from build123d import *

# Parameters (mm, degrees)
SKETCH1_R               = 12.7
BOSS_EXTRUDE1_DEPTH     = 36.83
SKETCH3_R               = 6.35
CUT_EXTRUDE1_DEPTH      = 18.415
CUT_EXTRUDE2_REACH      = 42.976
SKETCH4_R               = 6
CUT_EXTRUDE3_DEPTH      = 18.415
BOSS_EXTRUDE2_DEPTH     = 18.415
CUT_EXTRUDE6_DEPTH      = 18.415
CUT_EXTRUDE4_REACH      = 42.976
CUT_EXTRUDE4_END_RADIUS = 12.7
SKETCH6_R               = 1.5


with BuildPart() as part:
    # Sketch1 → Boss-Extrude1 (new body)
    with BuildSketch(Plane(origin=(0, 0, 0), x_dir=(1, 0, 0), z_dir=(0, 1, 0))):
        with Locations(Location((0, 0, 0), (0, 0, 270))):
            Circle(SKETCH1_R)
    extrude(amount=BOSS_EXTRUDE1_DEPTH)

    # Sketch3 → Cut-Extrude1 (cut)
    with BuildSketch(Plane(origin=(0, 0, 0), x_dir=(-1, 0, 0), z_dir=(0, -1, 0))):
        with Locations(Location((0, 0, 0), (0, 0, 90))):
            Circle(SKETCH3_R)
    extrude(amount=-CUT_EXTRUDE1_DEPTH, mode=Mode.SUBTRACT)

    # Sketch4 → Cut-Extrude2 (cut, up to next)
    with BuildSketch(Plane(origin=(0, 36.83, 0), x_dir=(1, 0, 0), z_dir=(0, 1, 0)), mode=Mode.PRIVATE) as cut_extrude2_sk1:
        with Locations(Location((0, 0, 0), (0, 0, 270))):
            Circle(SKETCH4_R)
    cut_extrude2_tool1 = extrude(cut_extrude2_sk1.sketch, amount=-CUT_EXTRUDE2_REACH, mode=Mode.PRIVATE) & part.part
    add(cut_extrude2_tool1.solids().sort_by_distance((0, 36.83, 0))[0], mode=Mode.SUBTRACT)

    # Sketch5 → Cut-Extrude3 (cut)
    with BuildSketch(Plane(origin=(0, 36.83, 0), x_dir=(1, 0, 0), z_dir=(0, 1, 0))):
        with BuildLine():
            Line((0, 8.032), (-2.0066, 8.032))
            Line((-2.0066, 8.032), (-2.0066, 5.654516464))
            ThreePointArc((-2.0066, 5.654516464), (0, 6), (2.0066, 5.654516464))
            Line((2.0066, 5.654516464), (2.0066, 8.032))
            Line((2.0066, 8.032), (0, 8.032))
        make_face()
    extrude(amount=-CUT_EXTRUDE3_DEPTH, mode=Mode.SUBTRACT)

    # Sketch9 → Boss-Extrude2 (add)
    with BuildSketch(Plane(origin=(0, 0, 0), x_dir=(-1, 0, 0), z_dir=(0, -1, 0))):
        with BuildLine():
            Line((3.274763384, 5.440443436), (6.348943915, 0.115806564))
            ThreePointArc((6.348943915, 0.115806564), (5.499261314, 3.175), (3.274763384, 5.440443436))
        make_face()
        with BuildLine():
            ThreePointArc((3.274763384, -5.440443436), (5.499261314, -3.175), (6.348943915, -0.115806564))
            Line((6.348943915, -0.115806564), (3.274763384, -5.440443436))
        make_face()
        with BuildLine():
            ThreePointArc((-3.074180531, -5.55625), (0, -6.35), (3.074180531, -5.55625))
            Line((3.074180531, -5.55625), (-3.074180531, -5.55625))
        make_face()
        with BuildLine():
            ThreePointArc((-6.348943915, -0.115806564), (-5.499261314, -3.175), (-3.274763384, -5.440443436))
            Line((-3.274763384, -5.440443436), (-6.348943915, -0.115806564))
        make_face()
        with BuildLine():
            Line((-6.348943915, 0.115806564), (-3.274763384, 5.440443436))
            ThreePointArc((-3.274763384, 5.440443436), (-5.499261314, 3.175), (-6.348943915, 0.115806564))
        make_face()
        with BuildLine():
            Line((-3.074180531, 5.55625), (3.074180531, 5.55625))
            ThreePointArc((3.074180531, 5.55625), (0, 6.35), (-3.074180531, 5.55625))
        make_face()
    extrude(amount=-BOSS_EXTRUDE2_DEPTH)

    # Sketch9<3> → Cut-Extrude6 (cut)
    with BuildSketch(Plane(origin=(0, 0, 0), x_dir=(-1, 0, 0), z_dir=(0, -1, 0))):
        with BuildLine():
            Line((-3.207902433, -5.55625), (-3.074180531, -5.55625))
            ThreePointArc((-3.074180531, -5.55625), (-3.175, -5.499261314), (-3.274763384, -5.440443436))
            Line((-3.274763384, -5.440443436), (-3.207902433, -5.55625))
        make_face()
        with BuildLine():
            ThreePointArc((-6.348943915, -0.115806564), (-6.35, 0), (-6.348943915, 0.115806564))
            Line((-6.348943915, 0.115806564), (-6.415804866, 0))
            Line((-6.415804866, 0), (-6.348943915, -0.115806564))
        make_face()
        with BuildLine():
            ThreePointArc((-3.274763384, 5.440443436), (-3.175, 5.499261314), (-3.074180531, 5.55625))
            Line((-3.074180531, 5.55625), (-3.207902433, 5.55625))
            Line((-3.207902433, 5.55625), (-3.274763384, 5.440443436))
        make_face()
        with BuildLine():
            ThreePointArc((3.074180531, 5.55625), (3.175, 5.499261314), (3.274763384, 5.440443436))
            Line((3.274763384, 5.440443436), (3.207902433, 5.55625))
            Line((3.207902433, 5.55625), (3.074180531, 5.55625))
        make_face()
        with BuildLine():
            Line((6.348943915, -0.115806564), (6.415804866, 0))
            Line((6.415804866, 0), (6.348943915, 0.115806564))
            ThreePointArc((6.348943915, 0.115806564), (6.349735973, 0.05790569), (6.35, 0))
            ThreePointArc((6.35, 0), (6.349735973, -0.05790569), (6.348943915, -0.115806564))
        make_face()
        with BuildLine():
            Line((3.207902433, -5.55625), (3.274763384, -5.440443436))
            ThreePointArc((3.274763384, -5.440443436), (3.175, -5.499261314), (3.074180531, -5.55625))
            Line((3.074180531, -5.55625), (3.207902433, -5.55625))
        make_face()
    extrude(amount=-CUT_EXTRUDE6_DEPTH, mode=Mode.SUBTRACT)

    # Cut-Extrude4: up to this cylinder (the profile starts inside it)
    cut_extrude4_end = Plane(origin=(0, 18.415, 0), z_dir=(0, -1, 0)) * Cylinder(CUT_EXTRUDE4_END_RADIUS, 136.482, mode=Mode.PRIVATE)
    # Sketch6 → Cut-Extrude4 (cut, up to the surface)
    with BuildSketch(Plane.XY, mode=Mode.PRIVATE) as cut_extrude4_sk1:
        with Locations((0, 30.48)):
            Circle(SKETCH6_R)
    cut_extrude4_tool1 = extrude(cut_extrude4_sk1.sketch, amount=-CUT_EXTRUDE4_REACH, mode=Mode.PRIVATE) & cut_extrude4_end
    add(cut_extrude4_tool1.solids().sort_by_distance((0, 30.48, 0))[0], mode=Mode.SUBTRACT)
    # Sketch6 → Cut-Extrude4 (cut, up to the surface)
    with BuildSketch(Plane.XY, mode=Mode.PRIVATE) as cut_extrude4_sk2:
        with Locations((0, 6.35)):
            Circle(SKETCH6_R)
    cut_extrude4_tool2 = extrude(cut_extrude4_sk2.sketch, amount=-CUT_EXTRUDE4_REACH, mode=Mode.PRIVATE) & cut_extrude4_end
    add(cut_extrude4_tool2.solids().sort_by_distance((0, 6.35, 0))[0], mode=Mode.SUBTRACT)


solid = part.part
Work out the finished part from the listing and answer in its coordinate system (mm). A direction names the side the tool comes from. Coordinates: 2 decimals unless noted, no trailing zeros. Loops run counter-clockwise (first coordinate to the right, second up) from the corner with the lowest first, then second, coordinate; pieces in that order, holes last. Notation, with made-up numbers: M 41.5,56 L 75.5,56 A27 cw 75.5,75 Z; hole C -31.75,-3.5 d2. An arc over 180 degrees is marked long. Answer in a Markdown table with one row per item. Add a question column.
1. Flat-ended cylindrical pins translate along their axes: P1, Ø1.8, axis at x = 4.5, z = -2, coming from the +Y side (3 decimals); P2, Ø1.5, axis at x = -3, z = 2, coming from the +Y side; P3, Ø1.5, axis at y = 11, z = -8, coming from the -X side; P4, Ø1.5, axis at y = 18, z = 1.5, coming from the -X side. Find the tip coordinate at first contact, or state that the pin passes through.
2. Find section D-D, the plane y = 6.35. Write down the section's boundary in (x, z).
3. Consider L1, parallel to Y at x = 0, z = -9.5; L2, parallel to X at y = 25, z = 0; L3, parallel to Z at x = 1.5, y = 19. Determine where each line is inside the solid, lowest interval first.
4. The mould has two halves that part along Z. Classify faces 4 (the cylindrical face through (-0.325, 4.886, -9.078)), 5 (the flat face through (-5, 18.415, -3)): pulls with the +Z half, pulls with the -Z half, needs draft (parallel to the pull), parting line crosses it, or undercut.
5. Find section C-C, the plane z = -8.5. Write down the section's boundary in (x, y).
6. Find section A-A, the plane y = 13.5. Write down the section's boundary in (x, z), then the cut area to 3 significant figures.
7. A tool of negligible diameter and unlimited length cuts with its end or side. For faces 1 (the flat face through (0, 18.415, -7)), 2 (the flat face through (3.08, 18.415, -5.33)), 3 (the cylindrical face through (-0.325, 29.016, -10.333)), from which of +Z, -Z, +X, -X, +Y, -Y can it reach the whole face along a straight path? Write none if from no direction.
8. Find section B-B, the plane x = -4.5. Write down the section's boundary in (y, z) (3 decimals).
Reported:
| question | item | result |
|---|---|---|
| 1 | P1 | stops at y = 18.415 |
| 1 | P2 | passes through |
| 1 | P3 | stops at x = -10.43 |
| 1 | P4 | stops at x = -12.68 |
| 2 | outline | M -6.42,0 L -3.21,5.56 L 3.21,5.56 L 6.42,0 L 3.21,-5.56 L 1.5,-5.56 L 1.5,-12.61 A12.7 ccw long -1.5,-12.61 L -1.5,-5.56 L -3.21,-5.56 Z |
| 3 | L1 | y = 0 to 4.85, 7.85 to 28.98, 31.98 to 36.83 |
| 3 | L2 | x = -12.7 to -6, 6 to 12.7 |
| 3 | L3 | z = -12.61 to -8.03, 5.81 to 12.61 |
| 4 | face 4 | needs draft |
| 4 | face 5 | undercut |
| 5 | outline | M -9.44,0 L 9.44,0 L 9.44,36.83 L -9.44,36.83 Z; hole C 0,6.35 d3; hole C 0,30.48 d3 |
| 6 | outline | C 0,0 d25.4; hole M -6.42,0 L -3.21,-5.56 L 3.21,-5.56 L 6.42,0 L 3.21,5.56 L -3.21,5.56 Z |
| 6 | area | 400 mm^2 |
| 7 | face 1 | +Y |
| 7 | face 2 | -Y |
| 7 | face 3 | -Z |
| 8 | outline | M 0,-11.876 L 36.83,-11.876 L 36.83,-3.969 L 18.415,-3.969 L 18.415,-3.318 L 0,-3.318 Z; M 0,3.318 L 18.415,3.318 L 18.415,3.969 L 36.83,3.969 L 36.83,11.876 L 0,11.876 Z |
